Build history of the part. All positions in model axes, mm. A direction names the side the tool comes from. Give positions to 0.01 mm unless a question says otherwise; leave off trailing zeros. Loops run counter-clockwise (first coordinate to the right, second up) from the corner with the lowest first, then second, coordinate; pieces in that order, holes last. Notation, with made-up numbers: (-36.5, -30) -> (5.5, -30) arc R27 cw to (5.5, -1) -> close; hole circle Ø6 at (9, -26.75). An arc over 180 degrees is marked (long way). Answer as a JSON object with one key per item and string values. Group by question number.
Q1. Band-saw the part on B-B, the plane x = 56. Write the cut outline in (y, z).
Q2. Tool access for faces 1 (the flat face through (10, -4.3, 22.4)), 2 (the flat face through (3.7, -36, 2)), 3 (the flat face through (6, -25, -17)): list every direction of +Z, -Z, +X, -X, +Y, -Y with a clear straight run to the whole face (end or side of a thin tool).
Q3. Wall check: probe 1 along Y at (x, z) = (3, 0); probe 2 along Y at (x, z) = (5.4, 0); probe 3 along Y at (x, z) = (7.25, -26). Give the ranges that are in metal, low to high. Write a range as from..to.
Q4. Drop flat-ended pins along their axis: pin 1 (4 mm diameter, centred on x = 103, y = 10, fed in from +Z); pin 2 (4 mm diameter, centred on y = 13.5, z = 34, fed in from +X); pin 3 (4 mm diameter, centred on x = 122.5, y = 5.5, fed in from +Z). Give the stop position or say it passes through.
Q5. Two-plate mould, pull along Y, no slides. Class faces 4 (the cylindrical face through (29.72, -19.961, -10.382)), 5 (the cylindrical face through (6.2, 1.05, -22.66)), 6 (the flat face through (2.5, 0, 20)): pulls with the +Y half, pulls with the -Y half, needs draft (parallel to the pull), parting line crosses it, or undercut.
Q6. Band-saw the part on C-C, the plane z = 8. Count the separate pieces of the cut face and the enclosed holes in it, plus the area to 3 significant figures.
Q7. Band-saw the part on A-A, the plane y = 34. Write the cut outline in (x, z).
from build123d import *

# Parameters (mm, degrees)
SKETCH2_R               = 55
BOSS_EXTRUDE1_DEPTH     = 10
SKETCH3_R               = 22.5
BOSS_EXTRUDE2_DEPTH     = 40
SKETCH4_R               = 19
CUT_EXTRUDE1_DEPTH      = 93.466210045
CUT_EXTRUDE1_DEPTH_BACK = 93.466210045
SKETCH14_R              = 37.5
SKETCH14_R_2            = 30.5
CUT_EXTRUDE5_DEPTH      = 3
SKETCH15_R              = 38
SKETCH15_R_2            = 30
CUT_EXTRUDE6_DEPTH      = 4
SKETCH16_R              = 2.5
CUT_EXTRUDE7_DEPTH      = 93.466210045
SKETCH17_R              = 5
CUT_EXTRUDE8_DEPTH      = 3.7
SKETCH20_R              = 3.5
SKETCH20_R_2            = 3
CUT_EXTRUDE9_DEPTH      = 10
SKETCH21_R              = 3.5
SKETCH21_R_2            = 3
CUT_EXTRUDE10_DEPTH     = 10
SKETCH22_R              = 24
BOSS_EXTRUDE3_DEPTH     = 140
SKETCH23_R              = 20.5
CUT_EXTRUDE11_DEPTH     = 140
SKETCH25_R              = 103.972470389
CUT_EXTRUDE12_DEPTH     = 2.5


with BuildPart() as part:
    # Sketch2 → Boss-Extrude1 (new body)
    with BuildSketch(Plane(origin=(0, 0, 0), x_dir=(0, 0, -1), z_dir=(1, 0, 0))):
        Circle(SKETCH2_R)
    extrude(amount=BOSS_EXTRUDE1_DEPTH)

    # Sketch3 → Boss-Extrude2 (add)
    with BuildSketch(Plane(origin=(10, 0, 0), x_dir=(0, 0, -1), z_dir=(1, 0, 0))):
        Circle(SKETCH3_R)
    extrude(amount=BOSS_EXTRUDE2_DEPTH)

    # Sketch4 → Cut-Extrude1 (cut, two sides)
    with BuildSketch(Plane.ZY) as cut_extrude1_sk:
        Circle(SKETCH4_R)
    extrude(amount=CUT_EXTRUDE1_DEPTH, mode=Mode.SUBTRACT)
    extrude(cut_extrude1_sk.sketch, amount=-CUT_EXTRUDE1_DEPTH_BACK, mode=Mode.SUBTRACT)

    # Sketch14 → Cut-Extrude5 (cut)
    with BuildSketch(Plane.ZY):
        Circle(SKETCH14_R)
        Circle(SKETCH14_R_2, mode=Mode.SUBTRACT)
    extrude(amount=-CUT_EXTRUDE5_DEPTH, mode=Mode.SUBTRACT)

    # Sketch15 → Cut-Extrude6 (cut)
    with BuildSketch(Plane(origin=(10, 0, 0), x_dir=(0, 0, -1), z_dir=(1, 0, 0))):
        Circle(SKETCH15_R)
        Circle(SKETCH15_R_2, mode=Mode.SUBTRACT)
    extrude(amount=-CUT_EXTRUDE6_DEPTH, mode=Mode.SUBTRACT)

    # Sketch16 → Cut-Extrude7 (cut, through all)
    with BuildSketch(Plane.ZY):
        with Locations((0, 34)):
            Circle(SKETCH16_R)
        with Locations((0, -34)):
            Circle(SKETCH16_R)
    extrude(amount=-CUT_EXTRUDE7_DEPTH, mode=Mode.SUBTRACT)

    # Sketch17 → Cut-Extrude8 (cut)
    with BuildSketch(Plane.ZY):
        with Locations((0, -34)):
            Circle(SKETCH17_R)
        with Locations((0, 34)):
            Circle(SKETCH17_R)
    extrude(amount=-CUT_EXTRUDE8_DEPTH, mode=Mode.SUBTRACT)

    # Sketch20 → Cut-Extrude9 (cut)
    with BuildSketch(Plane.ZY):
        with Locations((-26, 0)):
            Circle(SKETCH20_R)
        with Locations((-25, -8)):
            Circle(SKETCH20_R_2)
        with Locations((-25, 8)):
            Circle(SKETCH20_R_2)
    extrude(amount=-CUT_EXTRUDE9_DEPTH, mode=Mode.SUBTRACT)

    # Sketch21 → Cut-Extrude10 (cut)
    with BuildSketch(Plane.ZY):
        with Locations((0, 45)):
            Circle(SKETCH21_R)
        with Locations((-8, 44)):
            Circle(SKETCH21_R_2)
        with Locations((8, 44)):
            Circle(SKETCH21_R_2)
    extrude(amount=-CUT_EXTRUDE10_DEPTH, mode=Mode.SUBTRACT)


with BuildPart() as body_2:
    # Sketch22 → Boss-Extrude3 (new body)
    with BuildSketch(Plane(origin=(60, 0, 0), x_dir=(0, 0, -1), z_dir=(1, 0, 0))):
        Circle(SKETCH22_R)
    extrude(amount=BOSS_EXTRUDE3_DEPTH)

    # Sketch23 → Cut-Extrude11 (cut)
    with BuildSketch(Plane(origin=(200, 0, 0), x_dir=(0, 0, -1), z_dir=(1, 0, 0))):
        Circle(SKETCH23_R)
    extrude(amount=-CUT_EXTRUDE11_DEPTH, mode=Mode.SUBTRACT)


    add(part.part)  # loft5 joins it to this body
    # loft up to a face of the part (loft5)
    loft([Face(Wire([body_2.edges().sort_by_distance((60, -17.495247058, 16.429130542))[0]])), Face(Wire([body_2.edges().sort_by_distance((50, -16.401794117, 15.402309883))[0]]))])

    # loft up to a face of the part (cut_loft1)
    loft([Face(Wire([body_2.edges().sort_by_distance((60, 14.943856862, 14.033215672))[0]])), Face(Wire([body_2.edges().sort_by_distance((50, 13.850403921, -13.006395013))[0]]))], mode=Mode.SUBTRACT)

    # Sketch25 → Cut-Extrude12 (cut)
    with BuildSketch(Plane.ZY):
        Circle(SKETCH25_R)
    extrude(amount=-CUT_EXTRUDE12_DEPTH, mode=Mode.SUBTRACT)


solid = body_2.part
Worked answers:
{
 "1": {"outline": "circle Ø46.8 at (0, 0); hole circle Ø39.8 at (0, 0)"},
 "2": {"face 1": "none", "face 2": "-X", "face 3": "+X"},
 "3": {"probe 1": "-55..-39, -29..-19, 19..29, 39..41.5, 48.5..55", "probe 2": "-55..-36.5, -31.5..-19, 19..31.5, 36.5..41.5, 48.5..55", "probe 3": "-48.47..-27.71, -14.97..-10.83, -5.17..-3.5, 3.5..5.17, 10.83..14.97, 27.71..48.47"},
 "4": {"pin 1": "z = 22.63", "pin 2": "x = 10", "pin 3": "z = 23.74"},
 "5": {"face 4": "parting line crosses it", "face 5": "undercut", "face 6": "needs draft"},
 "6": {"separate pieces": "3", "enclosed holes": "0", "area": "1,870 mm2"},
 "7": {"outline": "(2.5, -43.23) -> (10, -43.23) -> (10, -16.97) -> (6, -16.97) -> (6, -2.5) -> (3.7, -2.5) -> (3.7, -5) -> (3, -5) -> (3, -15.82) -> (2.5, -15.82) -> close; (2.5, 15.82) -> (3, 15.82) -> (3, 5) -> (3.7, 5) -> (3.7, 2.5) -> (6, 2.5) -> (6, 16.97) -> (10, 16.97) -> (10, 43.23) -> (2.5, 43.23) -> close"}
}
